Source: three-view drawing plus pictorial views. Frame: mm from the lowest corner of the part. Give positions to 0.01 mm unless a question says otherwise; leave off trailing zeros. Loops run counter-clockwise (first coordinate to the right, second up) from the corner with the lowest first, then second, coordinate; pieces in that order, holes last. Notation, with made-up numbers: (-3.75, -38) -> (13.25, -38) arc R10 cw to (13.25, -30) -> close; hole circle Ø9 at (9.5, 78.5). An arc over 180 degrees is marked (long way). Answer in a Markdown table with one row per item. Add a question column.
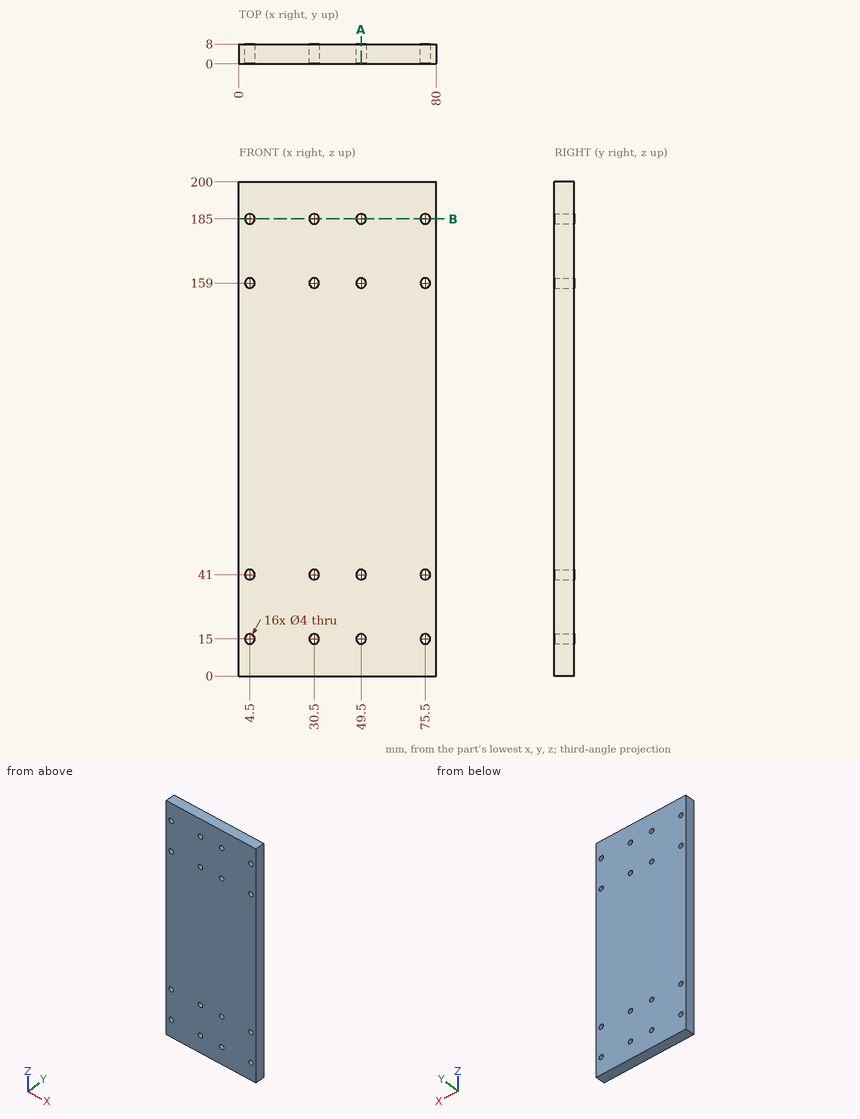
(1) Material intervals for line 1 along X through (y, z) = (2, 159); line 2 along Z through (x, y) = (49.5, 5.75); line 3 along Z through (x, y) = (74, 1.75), sorted ascending. Write a range as from..to.
(2) Cut plane A-A on x = 49.5. Return the cut outline in (y, z), then the cut area to 3 significant figures.
(3) Cut plane B-B on z = 185. Return the cut outline in (x, y).
(4) Pin query (flat end, axial travel): pin 1 Ø4.5 at (x, z) = (49.5, 15) entering from -Y. Return the tip coordinate at first contact, or that it passes through.
Answer list:
| question | item | result |
|---|---|---|
| 1 | line 1 | x = 0..2.5, 6.5..28.5, 32.5..47.5, 51.5..73.5, 77.5..80 |
| 1 | line 2 | z = 0..13, 17..39, 43..157, 161..183, 187..200 |
| 1 | line 3 | z = 0..13.68, 16.32..39.68, 42.32..157.68, 160.32..183.68, 186.32..200 |
| 2 | outline | (0, 0) -> (8, 0) -> (8, 13) -> (0, 13) -> close; (0, 17) -> (8, 17) -> (8, 39) -> (0, 39) -> close; (0, 43) -> (8, 43) -> (8, 157) -> (0, 157) -> close; (0, 161) -> (8, 161) -> (8, 183) -> (0, 183) -> close; (0, 187) -> (8, 187) -> (8, 200) -> (0, 200) -> close |
| 2 | area | 1,470 mm² |
| 3 | outline | (0, 0) -> (2.5, 0) -> (2.5, 8) -> (0, 8) -> close; (6.5, 0) -> (28.5, 0) -> (28.5, 8) -> (6.5, 8) -> close; (32.5, 0) -> (47.5, 0) -> (47.5, 8) -> (32.5, 8) -> close; (51.5, 0) -> (73.5, 0) -> (73.5, 8) -> (51.5, 8) -> close; (77.5, 0) -> (80, 0) -> (80, 8) -> (77.5, 8) -> close |
| 4 | pin 1 | stops at y = 0 |
